```python
from build123d import *

# Parameters (mm, degrees)
F0_W     = 262.7939805388
F0_H     = 60.3452790529
F1_DEPTH = 25.4
F3_DEPTH = 25.4
F4_W     = 30.9705659747
F4_H     = 9.5640197396
F5_DEPTH = 25.4
F6_R     = 10.4332897986
F6_R_2   = 5.6156262259
F7_DEPTH = 25.4


with BuildPart() as f1:
    # F0 (on Right) → F1 (new body)
    with BuildSketch(Plane.YZ):
        with Locations((42.1361811459, -43.3992138132)):
            Rectangle(F0_W, F0_H)
    extrude(amount=F1_DEPTH)

    # F2 (on face) → F3 (cut)
    with BuildSketch(Plane.YZ.offset(25.4)):
        with BuildLine():
            Line((7.4948265063, -30.0673552864), (-50.0055514276, -31.0259021828))
            ThreePointArc((-50.0055514276, -31.0259021828), (-62.7121802874, -44.1216826763), (-49.2391608491, -56.4276012088))
            Line((-49.2391608491, -56.4276012088), (8.1772062662, -54.1274810899))
            ThreePointArc((8.1772062662, -54.1274810899), (19.7263216343, -41.7601920363), (7.4948265063, -30.0673552864))
        make_face()
        with BuildLine():
            Line((144.9011948523, -28.0890673087), (88.3131250739, -29.3520299082))
            ThreePointArc((88.3131250739, -29.3520299082), (76.3994481978, -41.9242015804), (89.5937708362, -53.1449434175))
            Line((89.5937708362, -53.1449434175), (144.8779408269, -54.4762968558))
            ThreePointArc((144.8779408269, -54.4762968558), (158.3928280128, -41.2945819732), (144.9011948523, -28.0890673087))
        make_face()
    extrude(amount=-F3_DEPTH, mode=Mode.SUBTRACT)

    # F4 (on face) → F5 (cut)
    with BuildSketch(Plane.YZ.offset(25.4)):
        with Locations((45.589402318, -18.0085841566)):
            Rectangle(F4_W, F4_H)
    extrude(amount=-F5_DEPTH, mode=Mode.SUBTRACT)

    # F6 (on face) → F7 (cut)
    with BuildSketch(Plane.YZ.offset(25.4)):
        with Locations((-76.7875984311, -43.6257906258)):
            Circle(F6_R)
        with Locations((165.4747128487, -41.1704294384)):
            Circle(F6_R_2)
    extrude(amount=-F7_DEPTH, mode=Mode.SUBTRACT)


solid = f1.part
```
Geometry: final body of the model. Coordinates: model frame, mm. A direction names the side the tool comes from. Round coordinates to 2 decimals unless told otherwise and drop trailing zeros. Loops run counter-clockwise (first coordinate to the right, second up) from the corner with the lowest first, then second, coordinate; pieces in that order, holes last. Notation, with made-up numbers: (44, 81.25) -> (64, 81.25) arc R30 cw to (64, 105.25) -> close; hole circle Ø6 at (54.5, -35). An arc over 180 degrees is marked (long way). Write each question's results on one line, items separated by ' | '.
Item 1: Cut plane B-B on z = -38.5. Return the cut outline in (x, y), and give its area (3 significant figures).
Answers below:
outline: (0, -89.26) -> (25.4, -89.26) -> (25.4, -85.87) -> (0, -85.87) -> close; (0, -67.7) -> (25.4, -67.7) -> (25.4, -61.59) -> (0, -61.59) -> close; (0, 19.18) -> (25.4, 19.18) -> (25.4, 76.71) -> (0, 76.71) -> close; (0, 158.1) -> (25.4, 158.1) -> (25.4, 160.53) -> (0, 160.53) -> close; (0, 170.41) -> (25.4, 170.41) -> (25.4, 173.53) -> (0, 173.53) -> close | area: 1,840 mm²
Item 2: Pin query (flat end, axial travel): pin 1 Ø12.5 at (x, y) = (10.5, 39.5) entering from +Z. Return the tip coordinate at first contact, or that it passes through.
Answers below:
pin 1: stops at z = -22.79
Item 3: Cut plane A-A on y = 5. Return the cut outline in (x, z).
Answers below:
outline: (0, -73.57) -> (25.4, -73.57) -> (25.4, -54.25) -> (0, -54.25) -> close; (0, -30.11) -> (25.4, -30.11) -> (25.4, -13.23) -> (0, -13.23) -> close
Item 4: Set-up query: faces 1 (the face through (12.878, -62.718, -43.837)), 2 (the face through (13, 40, -73.572)), 3 (the face through (13, 61.075, -18)). Return all of +Z, -Z, +X, -X, +Y, -Y with unobstructed straight access to the full face (end or side cutting, diameter ignored); none if empty.
Answers below:
face 1: +X, -X | face 2: -Z, +X, -X, +Y, -Y | face 3: +Z, +X, -X
Item 5: Pull-direction query (Z, two-part tool) for faces 4 (the face through (25.4, 40, -43)), 5 (the face through (12.878, 76.388, -41.653)), 6 (the face through (13, 117, -13.227)); classes: pulls with the +Z half, pulls with the -Z half, needs draft (parallel to the pull), parting line crosses it, or undercut.
Answers below:
face 4: needs draft | face 5: undercut | face 6: pulls with the +Z half
Item 6: Cut plane D-D on y = 34. Return the cut outline in (x, z).
Answers below:
outline: (0, -73.57) -> (25.4, -73.57) -> (25.4, -22.79) -> (0, -22.79) -> close
Item 7: Cut plane C-C on x = 7.25. Return the cut outline in (y, z).
Answers below:
outline: (-89.26, -73.57) -> (173.53, -73.57) -> (173.53, -13.23) -> (61.07, -13.23) -> (61.07, -22.79) -> (30.1, -22.79) -> (30.1, -13.23) -> (-89.26, -13.23) -> close; hole circle Ø20.87 at (-76.79, -43.63); hole (-50.01, -31.03) arc R12.71 ccw (long way) to (-49.24, -56.43) -> (8.18, -54.13) arc R12.04 ccw to (7.49, -30.07) -> close; hole (88.31, -29.35) arc R11.93 ccw (long way) to (89.59, -53.14) -> (144.88, -54.48) arc R13.2 ccw (long way) to (144.9, -28.09) -> close; hole circle Ø11.23 at (165.47, -41.17)
Item 8: Line query: probe 1 along Y at (x, z) = (15, -35.5); probe 2 along Y at (x, z) = (22.5, -36.5); probe 3 along Y at (x, z) = (23, -44.5). Output: solid intervals per line, ascending. Write a range as [from, to].
Answers below:
probe 1: y = [-89.26, -83.33], [-70.24, -59.69], [17.76, 77.88], [157.06, 173.53] | probe 2: y = [-89.26, -84.41], [-69.17, -60.46], [18.35, 77.38], [157.5, 162.36], [168.59, 173.53] | probe 3: y = [-89.26, -87.18], [-66.39, -62.7], [19.49, 76.82], [157.99, 160.95], [170, 173.53]
